Check sheet for the modelled part. Datum: model origin and axes. Units: mm. A direction names the side the tool comes from. Round coordinates to 2 decimals unless told otherwise and drop trailing zeros. Answer as CSV lines item,"result". Start each with the question number.
from build123d import *

# Parameters (mm, degrees)
F5_T     = -5
F7_DEPTH = 40


with BuildPart() as f4:
    # F0 (on Top) → F4 section 0
    with BuildSketch(Plane.XY):
        Polygon((27.2798002192, 15.75), (0, 31.5), (-27.2798002192, 15.75), (-27.2798002192, -15.75), (0, -31.5), (27.2798002192, -15.75), align=None)
    # F2 (on offset) → F4 section 1
    with BuildSketch(Plane.XY.offset(20)):
        Polygon((-38.9711431703, -22.5), (0, -45), (38.9711431703, -22.5), (38.9711431703, 22.5), (0, 45), (-38.9711431703, 22.5), align=None)
    loft()

    # F5
    f5_openings = [f4.faces().sort_by_distance(p)[0] for p in [
        (0, 0, 20),
    ]]
    offset(amount=F5_T, openings=f5_openings)

    # F6 (on face) → F7 (join)
    with BuildSketch(Plane.XY.offset(20)):
        with BuildLine():
            Line((0, -38.3124026487), (-33.1795139738, -19.1562013243))
            Line((-33.1795139738, -19.1562013243), (-35.275328572, -20.3662204468))
            Line((-35.275328572, -20.3662204468), (-35.275328572, -18.7885692978))
            ThreePointArc((-35.275328572, -18.7885692978), (-36.075328572, -16.5781006622), (-36.875328572, -18.7885692978))
            Line((-36.875328572, -18.7885692978), (-36.875328572, -21.2899808775))
            Line((-36.875328572, -21.2899808775), (-38.9711431703, -22.5))
            Line((-38.9711431703, -22.5), (0, -45))
            Line((0, -45), (0, -42.579961755))
            Line((0, -42.579961755), (-2.1662859734, -41.3292559652))
            ThreePointArc((-2.1662859734, -41.3292559652), (-3.6806079661, -39.5312013243), (-1.3662859734, -39.9436153191))
            Line((-1.3662859734, -39.9436153191), (0, -40.7324408936))
            Line((0, -40.7324408936), (0, -38.3124026487))
        make_face()
        with BuildLine():
            Line((-35.275328572, 20.3662204468), (-33.1795139738, 19.1562013243))
            Line((-33.1795139738, 19.1562013243), (0, 38.3124026487))
            Line((0, 38.3124026487), (0, 40.7324408936))
            Line((0, 40.7324408936), (1.3662859734, 39.9436153191))
            ThreePointArc((1.3662859734, 39.9436153191), (3.6806079661, 39.5312013243), (2.1662859734, 41.3292559652))
            Line((2.1662859734, 41.3292559652), (0, 42.579961755))
            Line((0, 42.579961755), (0, 45))
            Line((0, 45), (-38.9711431703, 22.5))
            Line((-38.9711431703, 22.5), (-36.875328572, 21.2899808775))
            Line((-36.875328572, 21.2899808775), (-34.7090425987, 22.5406866674))
            ThreePointArc((-34.7090425987, 22.5406866674), (-32.394720606, 22.9531006622), (-33.9090425987, 21.1550460213))
            Line((-33.9090425987, 21.1550460213), (-35.275328572, 20.3662204468))
        make_face()
        with BuildLine():
            Line((33.1795139738, 19.1562013243), (33.1795139738, -19.1562013243))
            Line((33.1795139738, -19.1562013243), (35.275328572, -20.3662204468))
            Line((35.275328572, -20.3662204468), (33.9090425987, -21.1550460213))
            ThreePointArc((33.9090425987, -21.1550460213), (32.394720606, -22.9531006622), (34.7090425987, -22.5406866674))
            Line((34.7090425987, -22.5406866674), (36.875328572, -21.2899808775))
            Line((36.875328572, -21.2899808775), (38.9711431703, -22.5))
            Line((38.9711431703, -22.5), (38.9711431703, 22.5))
            Line((38.9711431703, 22.5), (36.875328572, 21.2899808775))
            Line((36.875328572, 21.2899808775), (36.875328572, 18.7885692978))
            ThreePointArc((36.875328572, 18.7885692978), (36.075328572, 16.5781006622), (35.275328572, 18.7885692978))
            Line((35.275328572, 18.7885692978), (35.275328572, 20.3662204468))
            Line((35.275328572, 20.3662204468), (33.1795139738, 19.1562013243))
        make_face()
    extrude(amount=F7_DEPTH)


solid = f4.part
1) Section check A-A on z = 35. Count the separate pieces of the cut face and the enclosed holes in it, then the cut area to 3 significant figures.
2) Mould release check, pull along Y, two halves, no side actions. Record for faces 6 (the face through (1.098, 41.946, 39.72)), 7 (the face through (-1.07, -41.96, 39.72)), 8 (the face through (33.18, 0, 40)): released by +Y, released by -Y, zero draft, split by the parting line, or undercut.
3) Access from +Z, -Z, +X, -X, +Y, -Y to the whole of each face (thin tool, end or side, straight path). Record for faces 1 (the face through (35.777, -21.924, 39.72)), 2 (the face through (36.875, 20, 40)), 3 (the face through (-34.24, 19.77, 39.72)), 4 (the face through (-3.7, -39.57, 39.72)), 5 (the face through (0, 44, 40)).
4) Material ranges on line 1 along X through (y, z) = (-19, 49.5); line 2 along X through (y, z) = (7, 29); line 3 along Z through (x, y) = (-2.5, 16.5), recorded low to high.
5) Depth check by flat-ended pin: pin 1 Ø2 at (x, y) = (36.08, 17.83) entering from +Z; pin 2 Ø1.2 at (y, z) = (-40, 39) entering from +X; pin 3 Ø3 at (y, z) = (20.5, 43) entering from -X. Enter the tip coordinate at first touch or a pass-through.
Solutions:
1,separate pieces,"3"
1,enclosed holes,"0"
1,area,"724 mm^2"
2,face 6,"released by +Y"
2,face 7,"undercut"
2,face 8,"zero draft"
3,face 1,"+Z, -Y"
3,face 2,"+Z, +Y"
3,face 3,"+Z, -X"
3,face 4,"+Z"
3,face 5,"+Z, +X, +Y"
4,line 1,"x = -36.88 to -35.28, 33.18 to 38.97"
4,line 2,"x = 33.18 to 38.97"
4,line 3,"z = 0 to 5"
5,pin 1,"stops at z = 20"
5,pin 2,"stops at x = 0"
5,pin 3,"stops at x = -38.11"
